from build123d import *

# Parameters (mm, degrees)
BOSS_EXTRUDE1_DEPTH     = 120
SKETCH2_W               = 10
SKETCH2_H               = 50
BOSS_EXTRUDE2_DEPTH     = 50
SKETCH3_R               = 5
CUT_EXTRUDE1_DEPTH      = 200
FILLET1_R               = 10
SKETCH5_R               = 4
CUT_EXTRUDE2_DEPTH      = 200
SKETCH6_R               = 12.5
SKETCH6_R_2             = 5
BOSS_EXTRUDE3_DEPTH     = 20
CUT_EXTRUDE3_DEPTH      = 12.5
CUT_EXTRUDE3_DEPTH_BACK = 12.5
CUT_EXTRUDE3_START      = 100
SKETCH7_R               = 3


with BuildPart() as part:
    # Sketch1 → Boss-Extrude1 (new body)
    with BuildSketch(Plane.XY):
        Polygon((0, 0), (200, 0), (200, 150), (190, 150), (190, 10), (10, 10), (10, 150), (0, 150), align=None)
    extrude(amount=BOSS_EXTRUDE1_DEPTH)

    # Sketch2 → Boss-Extrude2 (add)
    with BuildSketch(Plane.XY.offset(120)):
        with Locations((5, 125)):
            Rectangle(SKETCH2_W, SKETCH2_H)
        with Locations((195, 125)):
            Rectangle(SKETCH2_W, SKETCH2_H)
    extrude(amount=BOSS_EXTRUDE2_DEPTH)

    # Sketch3 → Cut-Extrude1 (cut)
    with BuildSketch(Plane.ZY):
        with Locations(Location((145, 125, 0), (0, 0, 270))):
            Circle(SKETCH3_R)
    extrude(amount=-CUT_EXTRUDE1_DEPTH, mode=Mode.SUBTRACT)

    # Fillet1
    fillet1_edges = [part.edges().sort_by_distance(p)[0] for p in [
        (195, 150, 0),
        (5, 100, 120),
        (5, 100, 170),
        (5, 150, 170),
        (195, 100, 120),
        (195, 100, 170),
        (195, 150, 170),
        (5, 150, 0),
    ]]
    fillet(fillet1_edges, radius=FILLET1_R)

    # Sketch5 → Cut-Extrude2 (cut)
    with BuildSketch(Plane.ZY):
        with Locations(Location((62.084380241, 90, 0), (0, 0, 270))):
            Circle(SKETCH5_R)
    extrude(amount=-CUT_EXTRUDE2_DEPTH, mode=Mode.SUBTRACT)

    # Sketch6 → Boss-Extrude3 (add)
    with BuildSketch(Plane.XZ):
        with Locations(Location((100, 60, 0), (0, 0, 90))):
            Circle(SKETCH6_R)
        with Locations(Location((100, 60, 0), (0, 0, 270))):
            Circle(SKETCH6_R_2, mode=Mode.SUBTRACT)
    extrude(amount=BOSS_EXTRUDE3_DEPTH)

    # Sketch7 → Cut-Extrude3 (cut, two sides: drawn at the far end of the back side and taken through both)
    with BuildSketch(Plane(origin=(0, 0, 0), x_dir=(0, 0, -1), z_dir=(1, 0, 0)).offset(CUT_EXTRUDE3_START - CUT_EXTRUDE3_DEPTH_BACK)):
        with Locations((-60, -10)):
            Circle(SKETCH7_R)
    extrude(amount=CUT_EXTRUDE3_DEPTH + CUT_EXTRUDE3_DEPTH_BACK, mode=Mode.SUBTRACT)


solid = part.part
Verification items for the finished model (mm, model axes). A direction names the side the tool comes from. Round coordinates to 2 decimals unless told otherwise and drop trailing zeros. Loops run counter-clockwise (first coordinate to the right, second up) from the corner with the lowest first, then second, coordinate; pieces in that order, holes last. Notation, with made-up numbers: (31, 44) - (51, 44) arc R20 cw to (51, 61) - close; hole circle Ø2 at (-31.5, 55.25). An arc over 180 degrees is marked (long way). Use one line per item in the form item = value.
1. Draft check along Z on faces 4 (the cylindrical face through (4.93, 122.693, 140.564)), 5 (the cylindrical face through (111.09, -9.86, 65.77)), 6 (the flat face through (5, 150, 84)), 7 (the cylindrical face through (5.07, 97.15, 123.01)). Enter one of: pulls with the +Z half, pulls with the -Z half, needs draft (parallel to the pull), parting line crosses it, or undercut.
A:
face_4 = undercut
face_5 = parting line crosses it
face_6 = needs draft
face_7 = pulls with the +Z half
2. Scan lines: probe 1 along X at (y, z) = (122, 21); probe 2 along Z at (x, y) = (5.25, 90); probe 3 along Y at (x, z) = (24.5, 101.5). Record each from-to range of solid material in increasing order.
A:
probe_1 = 0 to 10, 190 to 200
probe_2 = 0 to 58.08, 66.08 to 120
probe_3 = 0 to 10
3. Section check D-D on z = 89.5. Record the cut outline in (x, y).
A:
outline = (0, 0) - (200, 0) - (200, 150) - (190, 150) - (190, 10) - (10, 10) - (10, 150) - (0, 150) - close
4. Section check A-A on y = 36. Record the cut outline in (x, z).
A:
outline = (0, 0) - (10, 0) - (10, 120) - (0, 120) - close; (190, 0) - (200, 0) - (200, 120) - (190, 120) - close
5. Section check C-C on x = 100. Record the cut outline in (y, z).
A:
outline = (-20, 47.5) - (0, 47.5) - (0, 0) - (10, 0) - (10, 120) - (0, 120) - (0, 72.5) - (-20, 72.5) - (-20, 65) - (0, 65) - (0, 55) - (-20, 55) - close
6. Gauge pin test, flat ends, axial feed: pin 1 Ø8 at (x, z) = (6, 139) entering from -Y; pin 2 Ø16 at (x, z) = (100, 60) entering from +Y; pin 3 Ø7 at (y, z) = (-10, 60) entering from -X. Record the tip position at first contact, or that the pin passes through.
A:
pin_1 = 100
pin_2 = 10
pin_3 = 87.5
7. Section check B-B on y = 125. Record the cut outline in (x, z), and give its area (3 significant figures).
A:
outline = (0, 0) - (10, 0) - (10, 140) - (0, 140) - close; (0, 150) - (10, 150) - (10, 170) - (0, 170) - close; (190, 0) - (200, 0) - (200, 140) - (190, 140) - close; (190, 150) - (200, 150) - (200, 170) - (190, 170) - close
area = 3,200 mm²
8. Access from +Z, -Z, +X, -X, +Y, -Y to the whole of each face (thin tool, end or side, straight path). Record for faces 1 (the flat face through (10, 79, 65)), 2 (the flat face through (195, 100, 145)), 3 (the flat face through (100, 0, 60)).
A:
face_1 = +Z, -Z, +Y
face_2 = +Z, +X, -X, -Y
face_3 = -Y
